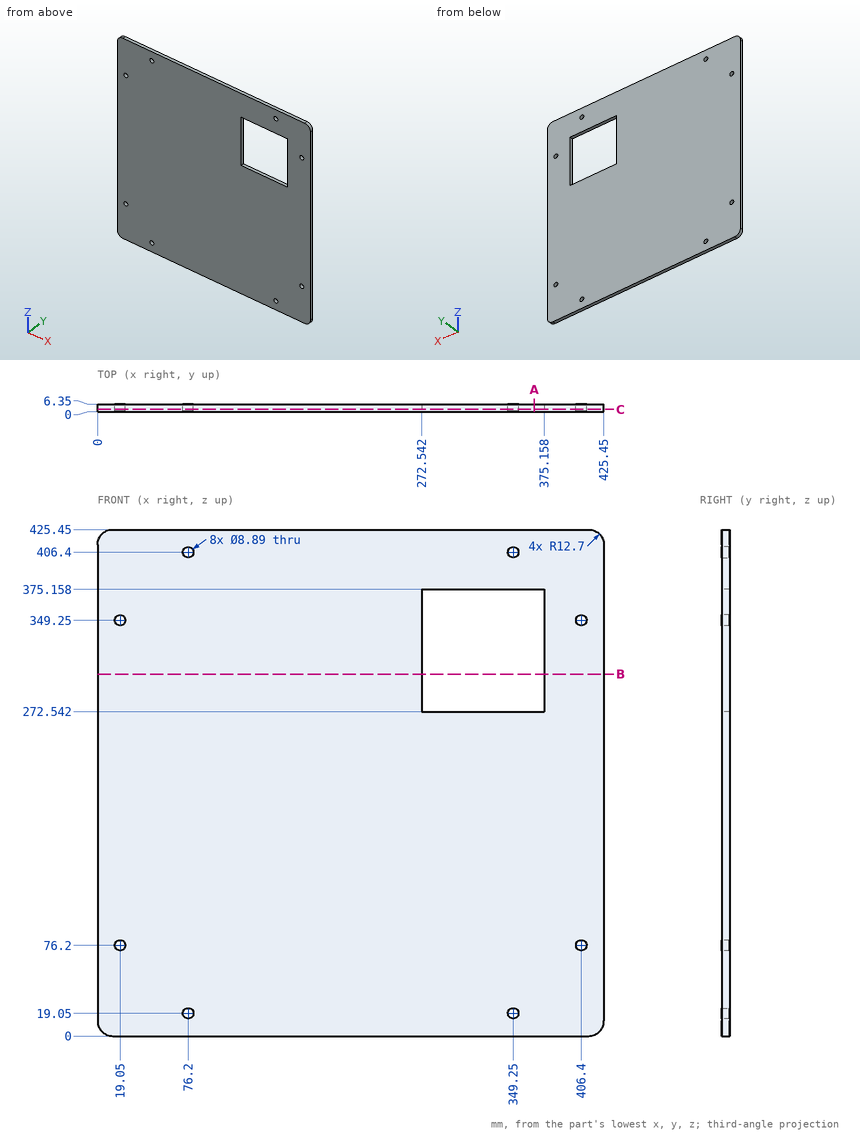
Input: dimensioned drawing with shaded views. Units: mm. Origin: part minimum x, y, z. Coordinates: 2 decimals unless noted, no trailing zeros. Order: outer loops, then holes, each group sorted by start corner. A loop starts at its lowest first (then second) coordinate and runs counter-clockwise, first axis right, second up. Notation, with made-up numbers: (-3, 48.5) -> (34, 48.5) arc R15 cw to (34, 62.5) -> close; hole circle Ø11 at (42.25, 4.5). An arc over 180 degrees is marked (long way). Answer in a Markdown table with one row per item.
Item 1: Ray query, L1, parallel to X at y = 2, z = 406.4 (3 decimals); L2, parallel to X at y = 2, z = 76.2 (3 decimals); L3, parallel to X at y = 2, z = 349.25 (3 decimals). Return the intervals inside material, ascending.
Return value:
| item | result |
|---|---|
| L1 | x = 0 to 71.755, 80.645 to 344.805, 353.695 to 425.45 |
| L2 | x = 0 to 14.605, 23.495 to 401.955, 410.845 to 425.45 |
| L3 | x = 0 to 14.605, 23.495 to 272.542, 375.158 to 401.955, 410.845 to 425.45 |
Item 2: Section B-B on z = 304. Output: boundary loops of the cut face in (x, y), plus the area to 3 significant figures.
Return value:
| item | result |
|---|---|
| outline | (0, 0) -> (272.54, 0) -> (272.54, 6.35) -> (0, 6.35) -> close; (375.16, 0) -> (425.45, 0) -> (425.45, 6.35) -> (375.16, 6.35) -> close |
| area | 2,050 mm² |
Item 3: Section C-C on y = 1.75. State how many separate pieces and enclosed holes the cut face has, plus the area to 3 significant figures.
Return value:
| item | result |
|---|---|
| separate pieces | 1 |
| enclosed holes | 9 |
| area | 170,000 mm² |
Item 4: Section A-A on x = 367. Output: boundary loops of the cut face in (y, z), plus the area to 3 significant figures.
Return value:
| item | result |
|---|---|
| outline | (0, 0) -> (6.35, 0) -> (6.35, 272.54) -> (0, 272.54) -> close; (0, 375.16) -> (6.35, 375.16) -> (6.35, 425.45) -> (0, 425.45) -> close |
| area | 2,050 mm² |
